Geometry: see drawing. Coordinates: mm, zero at the bounding-box minimum. Coordinates: 2 decimals unless noted, no trailing zeros. Loops run counter-clockwise (first coordinate to the right, second up) from the corner with the lowest first, then second, coordinate; pieces in that order, holes last.
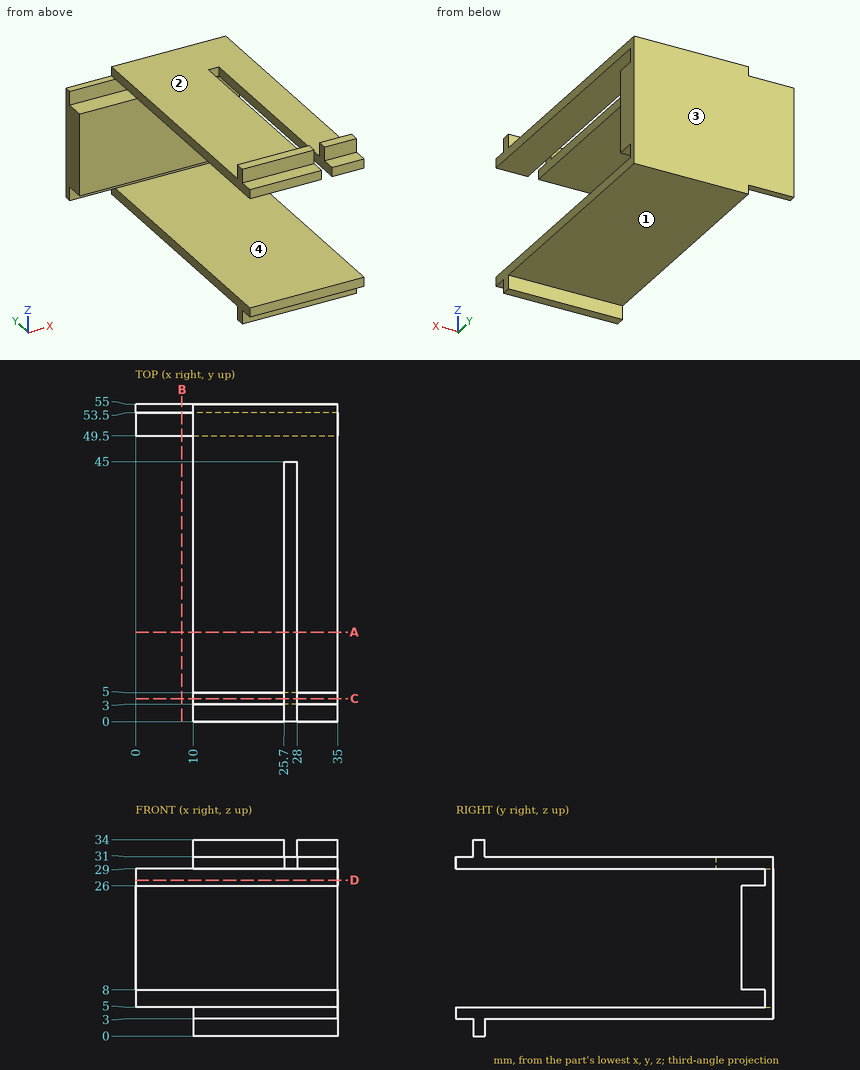
Item 1: Section query B-B (x = 8). Output: boundary loops of the cut face in (y, z).
Result:
outline: (49.5, 8) - (53.5, 8) - (53.5, 5) - (55, 5) - (55, 29) - (53.5, 29) - (53.5, 26) - (49.5, 26) - close
Item 2: Section query A-A (y = 15.5). Output: boundary loops of the cut face in (x, z), then the cut area to 3 significant figures.
Result:
outline: (10, 3) - (35, 3) - (35, 5) - (10, 5) - close; (10, 29) - (25.7, 29) - (25.7, 31) - (10, 31) - close; (28, 29) - (35, 29) - (35, 31) - (28, 31) - close
area: 95.4 mm2
Item 3: Line query: L1, parallel to Z at x = 19, y = 20; L2, parallel to X at y = 42, z = 30.5; L3, parallel to Y at x = 20.5, z = 14. Output: solid intervals per line, ascending.
Result:
L1: z = 3 to 5, 29 to 31
L2: x = 10 to 25.7, 28 to 35
L3: y = 49.5 to 55
Item 4: Mould query, pull axis Z, two halves, no side actions, for the marked faces 1, 2, 3 and 4. Classes: +Z half, -Z half, draft (parallel to the pull), parting line (faces both ways), or undercut.
Result:
face 1: -Z half
face 2: +Z half
face 3: draft
face 4: undercut
Item 5: Contact query for flat-ended pins moving along their axis: P1, Ø1.5, axis at x = 27.5, y = 1.5, coming from the -Z side; P2, Ø2.5, axis at x = 17, z = 1.5, coming from the -Y side; P3, Ø5, axis at x = 25.5, y = 46, coming from the +Z side; P4, Ø2.5, axis at y = 33.5, z = 32.5, coming from the -X side. Output: stop coordinate, or through.
Result:
P1: stops at z = 3
P2: stops at y = 3
P3: stops at z = 31
P4: passes through
Item 6: Section query C-C (y = 4). Output: boundary loops of the cut face in (x, z).
Result:
outline: (10, 0) - (35, 0) - (35, 5) - (10, 5) - close; (10, 29) - (25.7, 29) - (25.7, 34) - (10, 34) - close; (28, 29) - (35, 29) - (35, 34) - (28, 34) - close
Item 7: Section query D-D (z = 27). Output: boundary loops of the cut face in (x, y).
Result:
outline: (0, 53.5) - (35, 53.5) - (35, 55) - (0, 55) - close
